```python
from build123d import *

# Parameters (mm, degrees)
SALIENTE_EXTRUIR1_DEPTH    = 97.5
VACIADO1_T                 = -2
CORTAR_EXTRUIR1_DEPTH      = 146.020714686
CORTAR_EXTRUIR1_DEPTH_BACK = 146.020714686
CROQUIS2_W                 = 34
CROQUIS2_H                 = 22
CROQUIS5_W                 = 37
CROQUIS5_H                 = 15.5
SALIENTE_EXTRUIR3_DEPTH    = 22
CROQUIS7_R                 = 4.75
CORTAR_EXTRUIR2_DEPTH      = 22
VACIADO2_START             = 43
VACIADO2_OUTLINE_W         = 35
VACIADO2_OUTLINE_H         = 22
VACIADO2_OUTLINE_R         = 6.75
VACIADO2_DEPTH             = 11.5
CROQUIS9_W                 = 49.09
CROQUIS9_H                 = 20
CORTAR_EXTRUIR3_DEPTH      = 1
CROQUIS11_W                = 15
CROQUIS11_H                = 1
SALIENTE_EXTRUIR7_DEPTH    = 6
CROQUIS15_W                = 15
CROQUIS15_H                = 1
SALIENTE_EXTRUIR8_DEPTH    = 6


# Read off the part's stored shape, not the designer's step: Vaciado2
with BuildPart() as part:
    # Croquis1 → Saliente-Extruir1 (new body)
    with BuildSketch(Plane.XY):
        Polygon((0, 0), (94.998724665, 0), (94.998724665, 50), (35.998724665, 50), (35.998724665, 44.517964324), (11.046058241, 4.688773542), align=None)
    extrude(amount=SALIENTE_EXTRUIR1_DEPTH)

    # Vaciado1
    vaciado1_openings = [part.faces().sort_by_distance(p)[0] for p in [
        (65.498724665, 50, 48.75),
    ]]
    offset(amount=VACIADO1_T, openings=vaciado1_openings, kind=Kind.INTERSECTION)

    # Croquis2 → Cortar-Extruir1 (cut, two sides: drawn at the far end of the back side and taken through both)
    with BuildSketch(Plane(origin=(0, 50, 0), x_dir=(1, 0, 0), z_dir=(0, 1, 0)).offset(-CORTAR_EXTRUIR1_DEPTH_BACK)):
        with Locations((77.998724665, -11)):
            Rectangle(CROQUIS2_W, CROQUIS2_H)
        with Locations((77.998724665, -86.5)):
            Rectangle(CROQUIS2_W, CROQUIS2_H)
    extrude(amount=CORTAR_EXTRUIR1_DEPTH + CORTAR_EXTRUIR1_DEPTH_BACK, mode=Mode.SUBTRACT)

    # Croquis5 → Saliente-Extruir3 (add)
    with BuildSketch(Plane(origin=(0, 2, 0), x_dir=(1, 0, 0), z_dir=(0, 1, 0))):
        with Locations((74.498724665, -48.75)):
            Rectangle(CROQUIS5_W, CROQUIS5_H)
    extrude(amount=SALIENTE_EXTRUIR3_DEPTH)

    # Croquis7 → Cortar-Extruir2 (cut)
    with BuildSketch(Plane.XY.offset(56.5)):
        with Locations((82.778724665, 13.15)):
            Circle(CROQUIS7_R)
    extrude(amount=-CORTAR_EXTRUIR2_DEPTH, mode=Mode.SUBTRACT)

    # Vaciado2 outline → Vaciado2 (cut)
    with BuildSketch(Plane.XY.offset(VACIADO2_START)):
        with Locations((75.498724665, 13)):
            Rectangle(VACIADO2_OUTLINE_W, VACIADO2_OUTLINE_H)
        with Locations((82.778724665, 13.15)):
            Circle(VACIADO2_OUTLINE_R, mode=Mode.SUBTRACT)
    extrude(amount=VACIADO2_DEPTH, mode=Mode.SUBTRACT)

    # Croquis9 → Cortar-Extruir3 (cut)
    with BuildSketch(Plane(origin=(0, 2, 0), x_dir=(1, 0, 0), z_dir=(0, 1, 0))):
        with Locations((68.453724665, -32)):
            Rectangle(CROQUIS9_W, CROQUIS9_H)
        with Locations((68.453724665, -65.5)):
            Rectangle(CROQUIS9_W, CROQUIS9_H)
    extrude(amount=-CORTAR_EXTRUIR3_DEPTH, mode=Mode.SUBTRACT)

    # Croquis11 → Saliente-Extruir7 (add)
    with BuildSketch(Plane(origin=(0, 0, 95.5), x_dir=(-1, 0, 0), z_dir=(0, 0, -1))):
        with Locations((-45.498724665, 44.443211382)):
            Rectangle(CROQUIS11_W, CROQUIS11_H)
    extrude(amount=SALIENTE_EXTRUIR7_DEPTH)

    # Croquis15 → Saliente-Extruir8 (add)
    with BuildSketch(Plane.XY.offset(2)):
        with Locations((45.498724665, 44.44)):
            Rectangle(CROQUIS15_W, CROQUIS15_H)
    extrude(amount=SALIENTE_EXTRUIR8_DEPTH)


solid = part.part
```
Design review of the part built by this model. Coordinates are the model's own, in mm. A direction names the side the tool comes from. Coordinates: 2 decimals unless noted, no trailing zeros. Order: outer loops, then holes, each group sorted by start corner. A loop starts at its lowest first (then second) coordinate and runs counter-clockwise, first axis right, second up. Notation, with made-up numbers: M -38.75,43.5 L -6.75,43.5 A19 cw -6.75,71.5 Z; hole C 50.5,0 d5. An arc over 180 degrees is marked long. Answer as a JSON object with one key per item and string values. Group by question number.
1) For pin 1 (6 mm diameter, centred on y = 24.5, z = 51, fed in from -X); pin 2 (5 mm diameter, centred on x = 58, z = 84, fed in from +Y); pin 3 (3 mm diameter, centred on x = 47.5, z = 5.5, fed in from +Y); pin 4 (7.5 mm diameter, centred on x = 82.78, y = 13.15, fed in from -Z), all flat-tipped, find the tip position at first contact; note any pin that passes through.
2) Add section A-A, the plane y = 22. Write out the cut boundary in (x, z).
3) Add section B-B, the plane y = 13.15. Write out the cut boundary in (x, z).
4) Wall thickness on L1, parallel to X at y = 13, z = 51; L2, parallel to Z at x = 59.5, y = 46.5; L3, parallel to Y at x = 18.5, z = 76.5: over which ranges is each line inside the solid? List them lowest first.
5) Mouldability with a two-part tool opening along Y and no side actions: class faces 1 (the flat face through (29, 2, 48)), 2 (the flat face through (25.38, 23.8, 48.1)), 3 (the flat face through (23.697, 24.882, 48.068)), 4 (the flat face through (35.999, 47, 48)) as pulls with the +Y half, pulls with the -Y half, needs draft (parallel to the pull), parting line crosses it, or undercut.
6) Tool access review of faces 5 (the flat face through (41, 21, 2)), 6 (the cylindrical face through (89.01, 10.56, 48.67)), 7 (the flat face through (46, 44.943, 93)): name each direction out of +Z, -Z, +X, -X, +Y, -Y from which nothing blocks a thin tool from reaching the whole face with its end or side.
7) Add section C-C, the plane x = 40. Write out the cut boundary in (y, z), then the cut area to 3 significant figures.
8) Add section D-D, the plane z = 63.5. Write out the cut boundary in (x, y).
Computed values:
{
 "1": {"pin 1": "stops at x = 21.58", "pin 2": "stops at y = 2", "pin 3": "stops at y = 44.94", "pin 4": "passes through"},
 "2": {"outline": "M 21.89,0 L 61,0 L 61,2 L 24.25,2 L 24.25,95.5 L 61,95.5 L 61,97.5 L 21.89,97.5 Z; M 56,41 L 93,41 L 93,22 L 95,22 L 95,75.5 L 93,75.5 L 93,56.5 L 56,56.5 Z; hole M 58,43 L 93,43 L 93,54.5 L 58,54.5 Z"},
 "3": {"outline": "M 16.35,0 L 61,0 L 61,2 L 18.71,2 L 18.71,95.5 L 61,95.5 L 61,97.5 L 16.35,97.5 Z; M 56,41 L 78.03,41 L 78.03,56.5 L 56,56.5 Z; M 87.53,41 L 93,41 L 93,22 L 95,22 L 95,75.5 L 93,75.5 L 93,56.5 L 87.53,56.5 Z; hole M 58,43 L 76.03,43 L 76.03,54.5 L 58,54.5 Z; hole M 89.53,43 L 93,43 L 93,54.5 L 89.53,54.5 Z"},
 "4": {"L1": "x = 16.25 to 18.61, 56 to 58, 76.03 to 78.03, 87.53 to 89.53, 93 to 95", "L2": "z = 0 to 2, 95.5 to 97.5", "L3": "y = 0 to 2, 12.82 to 16.59"},
 "5": {"face 1": "undercut", "face 2": "undercut", "face 3": "pulls with the +Y half", "face 4": "needs draft"},
 "6": {"face 5": "+X", "face 6": "none", "face 7": "+X, +Y"},
 "7": {"outline": "M 0,0 L 50,0 L 50,2 L 44.94,2 L 44.94,8 L 43.94,8 L 43.94,2 L 2,2 L 2,95.5 L 43.94,95.5 L 43.94,89.5 L 44.94,89.5 L 44.94,95.5 L 50,95.5 L 50,97.5 L 0,97.5 Z", "area": "399 mm^2"},
 "8": {"outline": "M 0,0 L 95,0 L 95,50 L 93,50 L 93,1 L 43.91,1 L 43.91,2 L 9.83,2 L 12.41,3.09 L 38,43.94 L 38,50 L 36,50 L 36,44.52 L 11.05,4.69 Z"}
}
